Part model, mm, in its own coordinate system. Face numbers are marked on the shaded views. A direction names the side the tool comes from. Give positions to 0.01 mm unless a question says otherwise; leave off trailing zeros. Write each loop counter-clockwise with the first axis right and the second up, starting at its lowest first coordinate (ties: lowest second). Pieces come first, ordered by that corner, then holes.
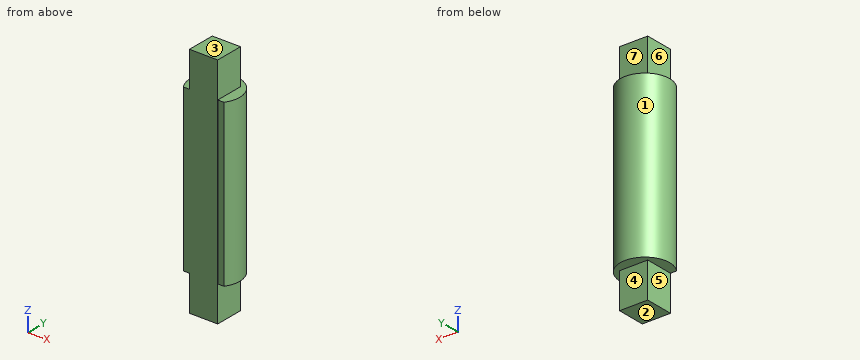
Autodesk Inventor part; units mm, degrees
ref_plane "Plano de trabajo2" through (-29.9, -16.92, 56) normal (0, 0, -1) x (0, 1, 0)
ref_plane "YZ Plane" through (0, 0, 0) normal (1, 0, 0) x (0, 1, 0)
ref_plane "XZ Plane" through (0, 0, 0) normal (0, 1, 0) x (-1, 0, 0)
sketch "Boceto1" plane through (0, 0, 0) normal (0, 1, 0) x (-1, 0, 0)
  line L0 (0, 0) -> (8, 0)
  line L1 (8, 0) -> (8, 66)
  line L2 (8, 66) -> (0, 66)
  line L3 (0, 66) -> (0, 0)
  dimension "d0" = 8
  dimension "d1" = 66
extrude "Extrusión1" add sketch "Boceto1" along normal blind 8
ref_plane "Plano de trabajo1" through (-12.4, 18.08, 10) normal (0, 0, 1) x (1, 0, 0)
sketch "Boceto2" plane through (-12.4, 18.08, 10) normal (0, 0, 1) x (1, 0, 0)
  line L0 (4.4, -18.08) -> (12.4, -18.08)
  line L1 (12.4, -18.08) -> (12.4, -10.08)
  line L2 (4.4, -10.08) -> (12.4, -10.08)
  line L3 (4.4, -18.08) -> (4.4, -10.08)
  line L4 (8.4, -18.08) -> (8.4, -7.08)
  circle A0 centre (8.4, -14.08) radius 7
  line L5 (4.4, -18.08) -> (2.6554, -18.08)
  line L6 (4.4, -18.08) -> (14.1617, -18.0553)
  point P0 (12.4, -18.0597)
  dimension "d4" = 11
ref_plane "Plano de trabajo2" through (-29.9, -16.92, 56) normal (0, 0, -1) x (0, 1, 0)
extrude "Extrusión2" add sketch "Boceto2" along normal up to surface (46 mm away) contours L6 L4 L0 | L5 A0 L4 L2 L3 | L3 L2 L4 L6 | L4 L6 L1 L0 | L4 L2 L1 L6 | L4 A0 L6 L1 L2
properties part number "Refuerzo bisagra"
1) Saw through at C-C (y = 9.75). Write the cut outline in (x, z), and give its area (3 significant figures).
Check result:
outline: (-7.99, 10) - (-0.01, 10) - (-0.01, 56) - (-7.99, 56) - close
area: 367 mm2
2) 3-axis set-ups, long thin cutter, end or side, ignore diameter. For the marked faces 4, 5, 6 and 7: which of +Z, -Z, +X, -X, +Y, -Y reach the whole face in a straight line?
Check result:
face 4: -Z, +X, -X, +Y
face 5: -Z, -X, +Y, -Y
face 6: +Z, -X, +Y, -Y
face 7: +Z, +X, -X, +Y
3) Saw through at A-A (y = 4). Write the cut outline in (x, z).
Check result:
outline: (-11, 10) - (-8, 10) - (-8, 0) - (0, 0) - (0, 10) - (3, 10) - (3, 56) - (0, 56) - (0, 66) - (-8, 66) - (-8, 56) - (-11, 56) - close
4) Saw through at B-B (x = -4). Write the cut outline in (y, z), and give its area (3 significant figures).
Check result:
outline: (0, 0) - (8, 0) - (8, 10) - (11, 10) - (11, 56) - (8, 56) - (8, 66) - (0, 66) - close
area: 666 mm2
5) Drill centre lines: L1, parallel to Z at x = -0.75, y = 8.5; L2, parallel to X at y = 3, z = 6.5; L3, parallel to Y at x = -5, z = 57.5. Where is each one in solid material? Low to high.
Check result:
L1: z = 10 to 56
L2: x = -8 to 0
L3: y = 0 to 8
6) Flat gauge pins, fed straight in: P1, Ø2.5, axis at y = 5.5, z = 29, coming from the +X side; P2, Ø6.5, axis at x = -5.5, z = 61.5, coming from the +Y side; P3, Ø2, axis at x = -1.5, y = 8, coming from the -Z side; P4, Ø6, axis at x = 1, z = 21, coming from the +Y side. Where does each tip first touch, or does it go through?
Check result:
P1: stops at x = 3
P2: stops at y = 8
P3: stops at z = 0
P4: stops at y = 10.71
7) Mould opens along Z. For the marked faces 1, 2 and 3 say: +Z half, -Z half, draft (parallel to the pull), parting line (faces both ways), or undercut.
Check result:
face 1: draft
face 2: -Z half
face 3: +Z half
